```python
from build123d import *

# Parameters (mm, degrees)
F0_W     = 60
F0_H     = 40
F1_DEPTH = 40
F3_DEPTH = 40
F5_DEPTH = 30
F7_DEPTH = 10


# Not quite as in the source:
# - ends of sketch curves that miss each other by under 0.0002 mm in the source are joined


with BuildPart() as f1:
    # F0 (on Front) → F1 (new body)
    with BuildSketch(Plane.XZ):
        with Locations((30, 20)):
            Rectangle(F0_W, F0_H)
    extrude(amount=F1_DEPTH)

    # F2 (on face) → F3 (cut)
    with BuildSketch(Plane.XY.offset(40)):
        with BuildLine():
            ThreePointArc((23.0189793024, -40), (3.0189805751, -19.9999993636), (23.0189805751, 0))
            Line((23.0189805751, 0), (0, 0))
            Line((0, 0), (0, -40))
            Line((0, -40), (23.0189793024, -40))
        make_face()
    extrude(amount=-F3_DEPTH, mode=Mode.SUBTRACT)

    # F4 (on face) → F5 (cut)
    with BuildSketch(Plane.XY.offset(40)):
        Polygon((50, 0), (33.0189805751, -40), (60, -40), (60, 0), align=None)
    extrude(amount=-F5_DEPTH, mode=Mode.SUBTRACT)

    # F6 (on face) → F7 (cut)
    with BuildSketch(Plane.XY.offset(40)):
        Polygon((40, 0), (23.0189805751, -40), (33.0189805751, -40), (50, 0), align=None)
    extrude(amount=-F7_DEPTH, mode=Mode.SUBTRACT)


solid = f1.part
```
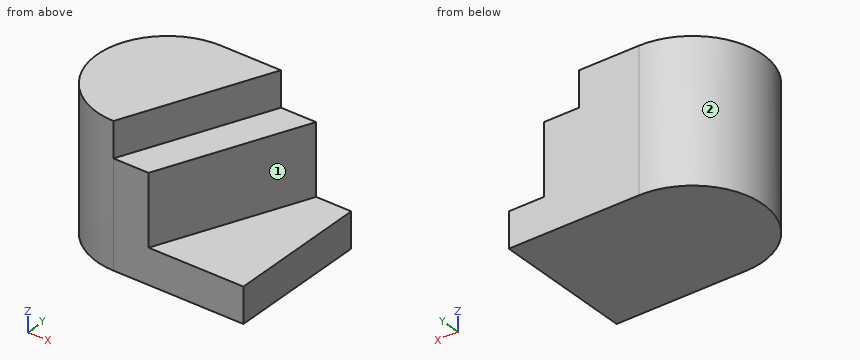
The listing builds one solid part. Answer for the finished solid, in the listing's coordinates (mm). Face numbers are marked on the shaded views. A direction names the side the tool comes from. Coordinates: 2 decimals unless noted, no trailing zeros. Write each loop counter-clockwise with the first axis right and the second up, starting at its lowest first coordinate (ties: lowest second). Pieces come first, ordered by that corner, then holes. Notation, with made-up numbers: (32, 24.5) - (86, 24.5) arc R17 cw to (86, 38.5) - close; hole circle Ø8 at (-7.5, 89). An arc over 180 degrees is marked (long way). Return JSON: item names as keys, results as strings. Group by question number.
1. A cutting plane is placed at A-A, the plane x = 35.5. Determine the outline of the cut face in (y, z).
2. A cutting plane is placed at C-C, the plane x = 29. Determine the outline of the cut face in (y, z).
3. Straight lines are drawn through the part: L1, parallel to Z at x = 44, y = -18.5; L2, parallel to Z at x = 39, y = -19.5; L3, parallel to X at y = -3, z = 12. For each, find the intervals that lie inside material, in ascending order.
4. Which of the six approach directions +Z, -Z, +X, -X, +Y, -Y give full straight-line access (tool end or side, diameter ignored) to the marked faces 1 and 2?
5. A cutting plane is placed at D-D, the plane x = 48.5. Determine the outline of the cut face in (y, z).
6. Given pin 1 (5 mm diameter, centred on y = -27.5, z = 16, fed in from +X); pin 2 (1.5 mm diameter, centred on x = 34, z = 34, fed in from -Y); pin 3 (12 mm diameter, centred on y = -15.5, z = 12, fed in from -X), each flat-ended and moving along its own axis, determine where each tip first touches the part or whether it passes through.
7. A cutting plane is placed at B-B, the plane y = -12. Determine the outline of the cut face in (x, z), plus the area to 3 significant figures.
Ans:
{
 "1": {"outline": "(-40, 0) - (0, 0) - (0, 40) - (-10.6, 40) - (-10.6, 30) - (-34.16, 30) - (-34.16, 10) - (-40, 10) - close"},
 "2": {"outline": "(-40, 0) - (0, 0) - (0, 40) - (-25.91, 40) - (-25.91, 30) - (-40, 30) - close"},
 "3": {"L1": "0 to 10", "L2": "0 to 30", "L3": "12.48 to 48.73"},
 "4": {"face 1": "+Z, +X, -Y", "face 2": "+Z, -Z, -X"},
 "5": {"outline": "(-40, 0) - (0, 0) - (0, 30) - (-3.53, 30) - (-3.53, 10) - (-40, 10) - close"},
 "6": {"pin 1": "x = 39.39", "pin 2": "y = -15.9", "pin 3": "x = 3.02"},
 "7": {"outline": "(4.69, 0) - (60, 0) - (60, 10) - (44.91, 10) - (44.91, 30) - (34.91, 30) - (34.91, 40) - (4.69, 40) - close", "area": "1,660 mm²"}
}
